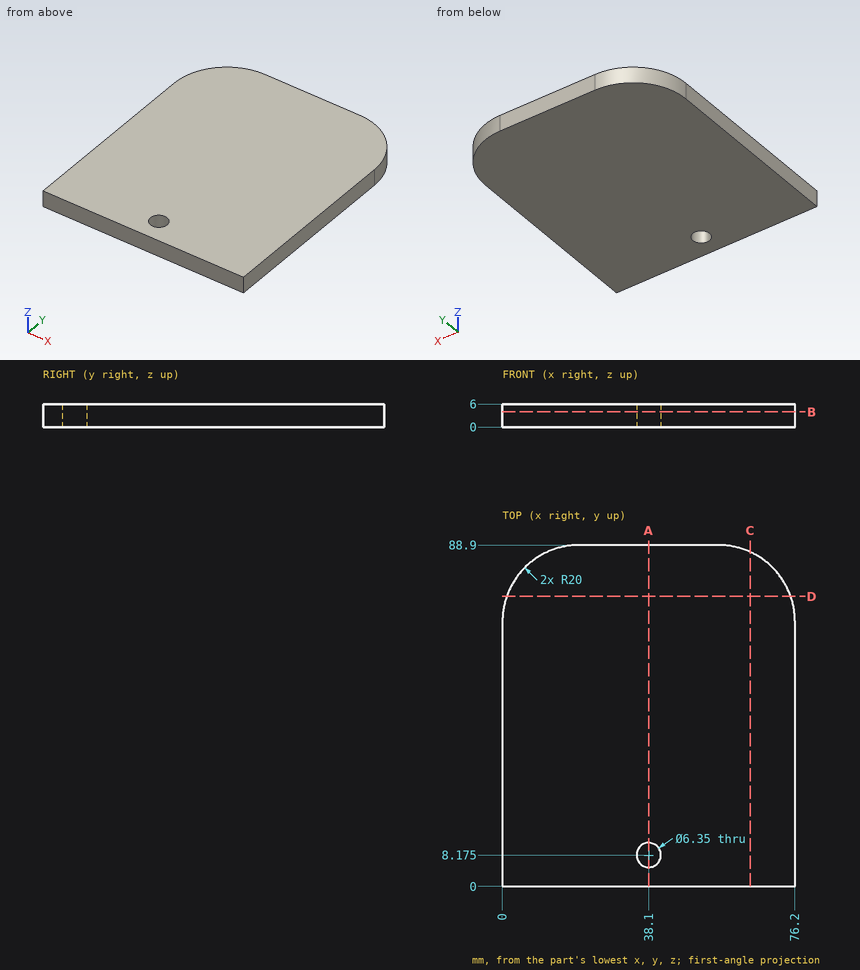
Verification items for this drawing (mm, ordinates from the low corner). Give positions to 0.01 mm unless a question says otherwise; leave off trailing zeros. Loops run counter-clockwise (first coordinate to the right, second up) from the corner with the lowest first, then second, coordinate; pieces in that order, holes last.
1. Cross-section at A-A on x = 38.1. Record the cut outline in (y, z), and give its area (3 significant figures).
Derived:
outline: (0, 0) - (5, 0) - (5, 6) - (0, 6) - close; (11.35, 0) - (88.9, 0) - (88.9, 6) - (11.35, 6) - close
area: 495 mm2
2. Cross-section at B-B on z = 3.95. Record the cut outline in (x, y) (3 decimals), and give its area (3 significant figures).
Derived:
outline: (0, 0) - (76.2, 0) - (76.2, 68.9) arc R20 ccw to (56.2, 88.9) - (20, 88.9) arc R20 ccw to (0, 68.9) - close; hole circle Ø6.35 at (38.1, 8.175)
area: 6,570 mm2
3. Go/stop test with flat-tipped pins: P1, Ø1.5, axis at y = 73.5, z = 1, coming from the -X side; P2, Ø5, axis at x = 38.1, y = 8.175, coming from the -Z side; P3, Ø2, axis at y = 76.5, z = 1.5, coming from the -X side. Record where each tip stops, or that it passes through.
Derived:
P1: stops at x = 0.37
P2: passes through
P3: stops at x = 1.12
4. Cross-section at D-D on y = 75.5. Record the cut outline in (x, z), and give its area (3 significant figures).
Derived:
outline: (1.12, 0) - (75.08, 0) - (75.08, 6) - (1.12, 6) - close
area: 444 mm2
5. Cross-section at C-C on x = 64.5. Record the cut outline in (y, z), and give its area (3 significant figures).
Derived:
outline: (0, 0) - (87.1, 0) - (87.1, 6) - (0, 6) - close
area: 523 mm2
6. Material ranges on probe 1 along Y at (x, z) = (38.1, 4.8); probe 2 along X at (y, z) = (7.5, 4.4); probe 3 along X at (y, z) = (6, 4.85), recorded low to high.
Derived:
probe 1: y = 0 to 5, 11.35 to 88.9
probe 2: x = 0 to 35, 41.2 to 76.2
probe 3: x = 0 to 35.79, 40.41 to 76.2
